```python
from build123d import *

# Parameters (mm, degrees)
F2_DEPTH       = 20
F3_DEPTH       = 22
F3_DEPTH_BACK  = 2
F1_W           = 29
F1_H           = 3
F7_DEPTH       = 22
F7_DEPTH_BACK  = 2
F5_W           = 6
F5_H           = 11.313708499
F4_W           = 6
F4_H           = 15
F6_W           = 6
F6_H           = 15
F8_DEPTH       = 2
F10_DEPTH      = 25
F12_DEPTH      = 5
F15_DEPTH      = 0.5
F16_R          = 16.2487088964
F16_R_2        = 9.9373882072
F17_DEPTH      = 2.5
F17_DEPTH_BACK = 2.5
F18_T4_DEPTH   = 31.116674808
F18_T9_DEPTH   = 19.1877426199
F18_T14_DEPTH  = 33.116674808
F18_T19_DEPTH  = 24.3595810189
F18_T24_DEPTH  = 24.3595810189
F18_T29_DEPTH  = 33.116674808
F18_T34_DEPTH  = 19.1877426199
F18_T39_DEPTH  = 31.116674808


# Not quite as in the source:
# - a fillet or chamfer that OpenCascade refuses, or shapes differently, is made with other operations: its cross-section is extruded or revolved along the edge and cut away or added
# - two fillets or chamfers of one size are made in one step


with BuildPart() as f2:
    # F1 (on Right) → F2 (new body)
    with BuildSketch(Plane.YZ):
        Polygon((-35, 30), (-35, 0), (-32, 0), (-32, 3), (-32, 27), (-9.2426406871, 27), (-3, 20.7573593129), (-3, 3), (-3, 0), (0, 0), (0, 22), (-8, 30), align=None)
    extrude(amount=F2_DEPTH)

    # F1 (on Right) → F3 (join, two sides)
    with BuildSketch(Plane.YZ) as f3_sk:
        Polygon((-32, 27), (-32, 3), (-3, 3), (-3, 20.7573593129), (-9.2426406871, 27), align=None)
    extrude(amount=F3_DEPTH)
    extrude(f3_sk.sketch, amount=-F3_DEPTH_BACK)

    # F1 (on Right) → F7 (join, two sides)
    with BuildSketch(Plane.YZ) as f7_sk:
        with Locations((-17.5, 1.5)):
            Rectangle(F1_W, F1_H)
    extrude(amount=F7_DEPTH)
    extrude(f7_sk.sketch, amount=-F7_DEPTH_BACK)

    # F5 (on face) + F4 (on face) + F6 (on face) → F8 (join)
    with BuildSketch(Plane(origin=(0, 11, 11), x_dir=(-1, 0, 0), z_dir=(0, 0.7071067812, 0.7071067812))):
        with Locations((-10, 21.2132034356)):
            Rectangle(F5_W, F5_H)
    with BuildSketch(Plane(origin=(0, 0, 0), x_dir=(-1, 0, 0), z_dir=(0, 1, 0))):
        with Locations((-10, 14.5)):
            Rectangle(F4_W, F4_H)
    with BuildSketch(Plane.XY.offset(30)):
        with Locations((10, -15.5)):
            Rectangle(F6_W, F6_H)
    extrude(amount=F8_DEPTH, dir=(0, 0.7071067812, 0.7071067812))

    # F9 (on face) → F10 (cut)
    with BuildSketch(Plane(origin=(-2, 0, 0), x_dir=(0, -1, 0), z_dir=(-1, 0, 0))):
        Polygon((22.18895033, -6.8113151938), (42.18895033, -6.8113151938), (42.18895033, 13.1886848062), (32.18895033, 13.1886848062), (32, 12.9997344762), (32, 0), (22.18895033, 0), align=None)
        Polygon((22.18895033, 3.1886848062), (22.18895033, 0), (32, 0), (32, 12.9997344762), align=None)
    extrude(amount=-F10_DEPTH, mode=Mode.SUBTRACT)

    # F11 (on face) → F12 (join)
    with BuildSketch(Plane(origin=(0, -9.5001327619, -9.5001327619), x_dir=(1, 0, 0), z_dir=(0, -0.7071067812, -0.7071067812))):
        Polygon((8, 26.8821576475), (8, 24.8821576475), (8, 22.8821576475), (12, 22.8821576475), (12, 24.8821576475), (12, 26.8821576475), align=None)
    extrude(amount=F12_DEPTH)

    # F11 (on face) → F13 (revolve)
    with BuildSketch(Plane(origin=(0, -9.5001327619, -9.5001327619), x_dir=(1, 0, 0), z_dir=(0, -0.7071067812, -0.7071067812))):
        Polygon((2, 28.8821576475), (2, 24.8821576475), (8, 24.8821576475), (8, 26.8821576475), (12, 26.8821576475), (12, 24.8821576475), (18, 24.8821576475), (18, 28.8821576475), align=None)
    revolve(axis=Axis((5, -27.094475165, 8.0942096412), (1, 0, 0)))

    # F14 (on face) → F15 (join)
    with BuildSketch(Plane(origin=(0, 1.4142135624, 0), x_dir=(-1, 0, 0), z_dir=(0, 1, 0))):
        with BuildLine():
            Line((-12, 21.4142135624), (-12, 10.4142135624))
            ThreePointArc((-12, 10.4142135624), (-11.7071067812, 9.7071067812), (-11, 9.4142135624))
            Line((-11, 9.4142135624), (-9, 9.4142135624))
            ThreePointArc((-9, 9.4142135624), (-8.2928932188, 9.7071067812), (-8, 10.4142135624))
            Line((-8, 10.4142135624), (-8, 21.4142135624))
            ThreePointArc((-8, 21.4142135624), (-8.2928932188, 22.1213203436), (-9, 22.4142135624))
            Line((-9, 22.4142135624), (-11, 22.4142135624))
            ThreePointArc((-11, 22.4142135624), (-11.7071067812, 22.1213203436), (-12, 21.4142135624))
        make_face()
    extrude(amount=F15_DEPTH)

    # F16 (on offset) → F17 (join, two sides)
    with BuildSketch(Plane.YZ.offset(10)) as f17_sk:
        with Locations((-42.5896607339, 38.0838625133)):
            Circle(F16_R)
        with Locations((-42.5896607339, 38.0838625133)):
            Circle(F16_R_2, mode=Mode.SUBTRACT)
    extrude(amount=F17_DEPTH)
    extrude(f17_sk.sketch, amount=-F17_DEPTH_BACK)

    # F18: chamfer of 2 x 1 on 8 edges, made by hand


with BuildPart() as f18_tool2:
    # F18_s3 → F18_t4 (new body)
    with BuildSketch(Plane.XY.offset(-5.1796577476)):
        Polygon((0, -3), (-2, -4), (-2, -3), align=None)
    extrude(amount=F18_T4_DEPTH)

    split(bisect_by=Plane.YZ, keep=Keep.BOTTOM)


with BuildPart() as f2_1:
    add(f2.part)

    # F18_t1: cut F18_tool2
    add(f18_tool2.part, mode=Mode.SUBTRACT)


with BuildPart() as f18_tool7:
    # F18_s8 → F18_t9 (new body)
    with BuildSketch(Plane(origin=(0, -8.2161085389, 8.2161085389), x_dir=(1, 0, 0), z_dir=(0, -0.7071067812, 0.7071067812))):
        Polygon((0, 12.5563491861), (-2, 11.5563491861), (-2, 12.5563491861), align=None)
    extrude(amount=F18_T9_DEPTH)

    split(bisect_by=Plane.YZ, keep=Keep.BOTTOM)


with BuildPart() as f2_2:
    add(f2_1.part)

    # F18_t6: cut F18_tool7
    add(f18_tool7.part, mode=Mode.SUBTRACT)


with BuildPart() as f18_tool12:
    # F18_s13 → F18_t14 (new body)
    with BuildSketch(Plane.XZ.offset(4.0629829395)):
        Polygon((0, 27), (-2, 26), (-2, 27), align=None)
    extrude(amount=F18_T14_DEPTH)

    split(bisect_by=Plane.YZ, keep=Keep.BOTTOM)


with BuildPart() as f2_3:
    add(f2_2.part)

    # F18_t11: cut F18_tool12
    add(f18_tool12.part, mode=Mode.SUBTRACT)


with BuildPart() as f18_tool17:
    # F18_s18 → F18_t19 (new body)
    with BuildSketch(Plane.XY.offset(32.1796577476)):
        Polygon((0, -32), (-2, -31), (-2, -32), align=None)
    extrude(amount=-F18_T19_DEPTH)

    split(bisect_by=Plane.YZ, keep=Keep.BOTTOM)


with BuildPart() as f2_4:
    add(f2_3.part)

    # F18_t16: cut F18_tool17
    add(f18_tool17.part, mode=Mode.SUBTRACT)


with BuildPart() as f18_tool22:
    # F18_s23 → F18_t24 (new body)
    with BuildSketch(Plane.XY.offset(7.8200767286)):
        Polygon((20, -32), (22, -31), (22, -32), align=None)
    extrude(amount=F18_T24_DEPTH)

    split(bisect_by=Plane.YZ.offset(20), keep=Keep.TOP)


with BuildPart() as f2_5:
    add(f2_4.part)

    # F18_t21: cut F18_tool22
    add(f18_tool22.part, mode=Mode.SUBTRACT)


with BuildPart() as f18_tool27:
    # F18_s28 → F18_t29 (new body)
    with BuildSketch(Plane.XZ.offset(4.0629829395)):
        Polygon((20, 27), (22, 26), (22, 27), align=None)
    extrude(amount=F18_T29_DEPTH)

    split(bisect_by=Plane.YZ.offset(20), keep=Keep.TOP)


with BuildPart() as f2_6:
    add(f2_5.part)

    # F18_t26: cut F18_tool27
    add(f18_tool27.part, mode=Mode.SUBTRACT)


with BuildPart() as f18_tool32:
    # F18_s33 → F18_t34 (new body)
    with BuildSketch(Plane(origin=(0, -8.2161085389, 8.2161085389), x_dir=(1, 0, 0), z_dir=(0, -0.7071067812, 0.7071067812))):
        Polygon((20, 12.5563491861), (22, 11.5563491861), (22, 12.5563491861), align=None)
    extrude(amount=F18_T34_DEPTH)

    split(bisect_by=Plane.YZ.offset(20), keep=Keep.TOP)


with BuildPart() as f2_7:
    add(f2_6.part)

    # F18_t31: cut F18_tool32
    add(f18_tool32.part, mode=Mode.SUBTRACT)


with BuildPart() as f18_tool37:
    # F18_s38 → F18_t39 (new body)
    with BuildSketch(Plane.XY.offset(25.9370170605)):
        Polygon((22, -4), (20, -3), (22, -3), align=None)
    extrude(amount=-F18_T39_DEPTH)

    split(bisect_by=Plane.YZ.offset(20), keep=Keep.TOP)


with BuildPart() as f2_8:
    add(f2_7.part)

    # F18_t36: cut F18_tool37
    add(f18_tool37.part, mode=Mode.SUBTRACT)


solid = f2_8.part
```
CAD build for the part. Positions are in the model's coordinates, mm. A direction names the side the tool comes from. Give positions to 0.01 mm unless a question says otherwise; leave off trailing zeros. Order: outer loops, then holes, each group sorted by start corner. A loop starts at its lowest first (then second) coordinate and runs counter-clockwise, first axis right, second up.
(1) Flat gauge pins, fed straight in: pin 1 (16 mm diameter, centred on y = -35, z = 43, fed in from +X); pin 2 (8 mm diameter, centred on x = 8, z = 32.5, fed in from +Y); pin 3 (1.6 mm diameter, centred on x = 9, z = 2.5, fed in from -Y). Where does each tip first touch, or does it go through?
(2) Saw through at B-B, the plane x = 0.75. Give the cut face in (y, z), then the cut area to 3 significant figures.
(3) Saw through at D-D, the plane y = -14. Give the cut face in (x, z).
(4) Saw through at A-A, the plane y = -38. Give the cut face in (x, z), then the cut area to 3 significant figures.
(5) Mould opens along Y. For faces 4 (the cylindrical face through (9.888, -31.086, 7.833)), 5 (the flat face through (12.7, 1.414, 16)), 6 (the flat face through (21, -20.5, 26.5)), 7 (the cylindrical face through (9.96, -50.48, 32.04)) say: released by +Y, released by -Y, zero draft, split by the parting line, or undercut.
(6) Drill centre lines: L1, parallel to Y at x = 17.5, z = 9; L2, parallel to Z at x = 10.25, y = -40.5; L3, parallel to X at y = -44.5, z = 27. Where is each one in solid material? Low to high.
(7) Tool access for faces 1 (the flat face through (16, -4, 26)), 2 (the flat face through (3, -4, 26)), 3 (the flat face through (18, -28, 7)): list every direction of +Z, -Z, +X, -X, +Y, -Y with a clear straight run to the whole face (end or side of a thin tool).
(8) Saw through at C-C, the plane z = 18.5. Give the cut face in (x, y), then the cut area to 3 significant figures.
Results found:
1. pin 1: stops at x = 12.5
1. pin 2: stops at y = -3.67
1. pin 3: stops at y = -29.37
2. outline: (-35, 13.19) - (-32.19, 13.19) - (-22.19, 3.19) - (-22.19, 0) - (0, 0) - (0, 22) - (-8, 30) - (-35, 30) - close
2. area: 899 mm2
3. outline: (-2, 0) - (22, 0) - (22, 26) - (20, 27) - (20, 30) - (13, 30) - (13, 31.41) - (7, 31.41) - (7, 30) - (0, 30) - (0, 27) - (-2, 26) - close
4. outline: (7.5, 22.5) - (12.5, 22.5) - (12.5, 29.27) - (7.5, 29.27) - close; (7.5, 46.9) - (12.5, 46.9) - (12.5, 53.67) - (7.5, 53.67) - close
4. area: 67.7 mm2
5. face 4: undercut
5. face 5: released by +Y
5. face 6: zero draft
5. face 7: undercut
6. L1: y = -30.99 to 0
6. L2: z = 21.97 to 28.37, 47.8 to 54.2
6. L3: x = 7.5 to 12.5
7. face 1: +Z, +X, +Y
7. face 2: +Z, -X, +Y
7. face 3: -Z, +X, -Y
8. outline: (-2, -31) - (0, -32) - (0, -35) - (20, -35) - (20, -32) - (22, -31) - (22, -4) - (20, -3) - (20, 0) - (13, 0) - (13, 1.41) - (12, 1.41) - (12, 1.91) - (8, 1.91) - (8, 1.41) - (7, 1.41) - (7, 0) - (0, 0) - (0, -3) - (-2, -4) - close
8. area: 822 mm2
